Here's how the part is built. I have some questions about the finished solid (model axes, mm). Round coordinates to 2 decimals unless told otherwise and drop trailing zeros. Order: outer loops, then holes, each group sorted by start corner. A loop starts at its lowest first (then second) coordinate and runs counter-clockwise, first axis right, second up. Notation, with made-up numbers: (-16, 34.25) - (-4, 34.25) arc R30 cw to (-4, 73.25) - close; hole circle Ø7 at (-37.75, 14). An arc over 180 degrees is marked (long way). One line per item, written item: value.
from build123d import *

# Parameters (mm, degrees)
SKETCH1_W           = 86
SKETCH1_H           = 16
BOSS_EXTRUDE1_DEPTH = 1.3
SKETCH2_W           = 1.4
SKETCH2_H           = 8
SKETCH2_W_2         = 30
SKETCH2_H_2         = 1.4
BOSS_EXTRUDE2_DEPTH = 1.3
CUT_EXTRUDE1_DEPTH  = 46.40275322
CUT_EXTRUDE2_DEPTH  = 46.40275322


with BuildPart() as part:
    # Sketch1 → Boss-Extrude1 (new body)
    with BuildSketch(Plane.XY):
        Rectangle(SKETCH1_W, SKETCH1_H)
    extrude(amount=BOSS_EXTRUDE1_DEPTH)

    # Sketch2 → Boss-Extrude2 (add)
    with BuildSketch(Plane.XY.offset(1.3)):
        with Locations((-43.7, 0.5)):
            Rectangle(SKETCH2_W, SKETCH2_H)
        with Locations((43.7, 0.5)):
            Rectangle(SKETCH2_W, SKETCH2_H)
        with Locations((0, -8.7)):
            Rectangle(SKETCH2_W_2, SKETCH2_H_2)
    extrude(amount=-BOSS_EXTRUDE2_DEPTH)

    # Sketch3 → Cut-Extrude1 (cut, through all)
    with BuildSketch(Plane.XY.offset(1.3)):
        with BuildLine():
            Line((-43, 8), (43, 8))
            ThreePointArc((43, 8), (0, 4.461913504), (-43, 8))
        make_face()
        Polygon((-20, 0), (-31.555732492, 3.872025984), (-33.777866246, 3.872025984), (-36, 0), align=None)
        Polygon((36, 0), (20, 0), (31.555732492, 3.872025984), (33.777866246, 3.872025984), align=None)
    extrude(amount=-CUT_EXTRUDE1_DEPTH, mode=Mode.SUBTRACT)

    # Sketch4 → Cut-Extrude2 (cut, through all)
    with BuildSketch(Plane.XY.offset(1.3)):
        Polygon((-13.931038069, 4.831038069), (-11.5, 2.4), (11.5, 2.4), (13.931038069, 4.831038069), align=None)
        with BuildLine():
            Line((-20, -5), (20, -5))
            add(Edge.make_bspline(
                [(20, -5), (20, -2), (0, -2), (-20, -2), (-20, -5)],
                knots=[0, 0, 0, 1.570796327, 1.570796327, 3.141592654, 3.141592654, 3.141592654], degree=2, weights=[1, 0.707106781, 1, 0.707106781, 1]))
        make_face()
    extrude(amount=-CUT_EXTRUDE2_DEPTH, mode=Mode.SUBTRACT)


solid = part.part
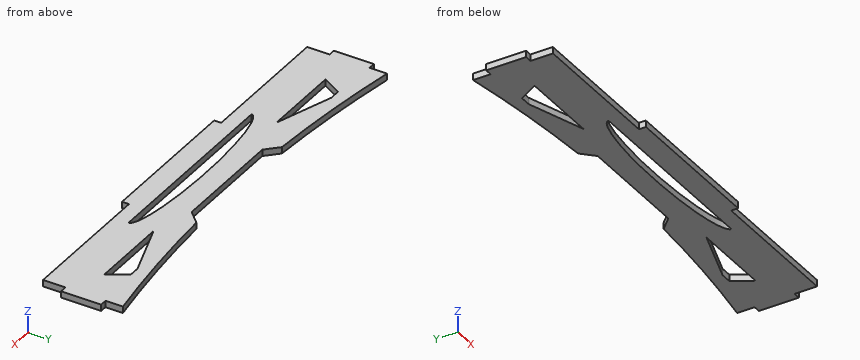
Q1. Will these pins go through, and if not, where does the flat tip stop? pin 1 (0.6 mm diameter, centred on y = 6, z = 0.5, fed in from -X); pin 2 (0.6 mm diameter, centred on x = -31, z = 0.5, fed in from +Y); pin 3 (0.6 mm diameter, centred on x = 32.5, z = 0.5, fed in from -Y); pin 4 (2 mm diameter, centred on x = -30.5, y = 2, fed in from +Z).
Results list:
pin 1: x = -43
pin 2: y = 6.33
pin 3: y = -8
pin 4: through
Q2. If I drill on line 1 along Y through (x, z) = (2, 0.25); line 2 along Y through (x, z) = (28, 0.45); line 3 along X through (y, z) = (-4, 0.3), over which ranges is the centre line in solid material (lowest first)?
Results list:
line 1: -9.4 to -5, -2.02 to 2.4
line 2: -8 to 0, 2.68 to 5.96
line 3: -43 to -18.86, 18.86 to 43
Q3. If we section it at A-A, the plane x = 21: Please give me the cut outline in (y, z).
Results list:
outline: (-8, 0) - (0, 0) - (0, 1.3) - (-8, 1.3) - close; (0.34, 0) - (5.3, 0) - (5.3, 1.3) - (0.34, 1.3) - close
Q4. If we section it at C-C, the plane x = -32.5: Please give me the cut outline in (y, z).
Results list:
outline: (-8, 0) - (0, 0) - (0, 1.3) - (-8, 1.3) - close; (3.87, 0) - (6.48, 0) - (6.48, 1.3) - (3.87, 1.3) - close
Q5. If we section it at B-B, the plane z = 0.5: Give the number of separate pieces and of enclosed holes in the cut face, then the cut area to 3 significant figures.
Results list:
separate pieces: 1
enclosed holes: 3
area: 1,020 mm²
